```python
from build123d import *

# Parameters (mm, degrees)
CYLINDER017_R     = 3.5
CYLINDER017_DEPTH = 4
CYLINDER015_R     = 1.65
CYLINDER015_DEPTH = 20
CYLINDER016_R     = 3.5
CYLINDER016_DEPTH = 4
CYLINDER014_R     = 1.65
CYLINDER014_DEPTH = 20
BOX001_W          = 95
BOX001_H          = 30
BOX001_DEPTH      = 5
CYLINDER010_R     = 24.8
CYLINDER010_DEPTH = 10


with BuildPart() as zylinder017:
    # Cylinder017 → Cylinder017 (new body)
    with BuildSketch(Plane.XY):
        Circle(CYLINDER017_R)
    extrude(amount=CYLINDER017_DEPTH)


with BuildPart() as screw02:
    # Cylinder015 → Cylinder015 (new body)
    with BuildSketch(Plane.XY):
        Circle(CYLINDER015_R)
    extrude(amount=CYLINDER015_DEPTH)

    # Fusion003: union Zylinder017
    add(zylinder017.part)


with BuildPart() as screw02_1:
    # Fusion003 placement: moved
    add(screw02.part.moved(Location((4, 57, 10))))


with BuildPart() as zylinder016:
    # Cylinder016 → Cylinder016 (new body)
    with BuildSketch(Plane.XY):
        Circle(CYLINDER016_R)
    extrude(amount=CYLINDER016_DEPTH)


with BuildPart() as compound002:
    # Cylinder014 → Cylinder014 (new body)
    with BuildSketch(Plane.XY):
        Circle(CYLINDER014_R)
    extrude(amount=CYLINDER014_DEPTH)

    # Fusion002: union Zylinder016
    add(zylinder016.part)


with BuildPart() as compound002_1:
    # Fusion002 placement: moved
    add(compound002.part.moved(Location((4, 38, 10))))

    # Compound002: union Screw02
    add(screw02_1.part)


with BuildPart() as obj1:
    # Box001 → Box001 (new body)
    with BuildSketch(Plane(origin=(0, 32.5, 10), x_dir=(1, 0, 0), z_dir=(0, 0, 1))):
        with Locations((47.5, 15)):
            Rectangle(BOX001_W, BOX001_H)
    extrude(amount=BOX001_DEPTH)


with BuildPart() as rotatingtable:
    # Cylinder010 → Cylinder010 (new body)
    with BuildSketch(Plane(origin=(47.5, 47.5, 0), x_dir=(1, 0, 0), z_dir=(0, 0, 1))):
        Circle(CYLINDER010_R)
    extrude(amount=CYLINDER010_DEPTH)

    # Fusion001: union obj1
    add(obj1.part)

    # Cut006: cut Compound002
    add(compound002_1.part, mode=Mode.SUBTRACT)


solid = rotatingtable.part
```
Could you check a few things on this model? Use its own coordinates, in mm. A direction names the side the tool comes from. Give positions to 0.01 mm unless a question says otherwise; leave off trailing zeros. Order: outer loops, then holes, each group sorted by start corner. A loop starts at its lowest first (then second) coordinate and runs counter-clockwise, first axis right, second up.
Q1. Suppose I cut it at C-C, the plane z = 13. Write out the boundary of the cut face in (x, y), and give its area (3 significant figures).
Q2. Suppose I cut it at D-D, the plane x = 47.5. Write out the boundary of the cut face in (y, z), and give its area (3 significant figures).
Q3. For faces 1 (the flat face through (47, 32.5, 12)), 2 (the flat face through (47, 62.5, 12)), 3 (the cylindrical face through (7.34, 58.05, 11.97)), 4 (the flat face through (47, 48, 15)), which set-ups out of +Z, -Z, +X, -X, +Y, -Y let a thin tool reach every point of the face, with its end or its side?
Q4. Suppose I cut it at A-A, the plane x = 4. Write out the boundary of the cut face in (y, z), and give its area (3 significant figures).
Q5. I'm going to push flat-ended pins straight in: P1, Ø14, axis at x = 10, y = 48.5, coming from the -Z side; P2, Ø3, axis at x = 38.5, y = 28.5, coming from the +Z side; P3, Ø4, axis at x = 40, z = 11.5, coming from the +Y side. Where does each tip first touch, or does it pass through?
Q6. Suppose I cut it at B-B, the plane y = 38. Write out the boundary of the cut face in (x, z), and give its area (3 significant figures).
Q7. If I drill on line 1 along Y through (x, z) = (4, 14.4); line 2 along X through (y, z) = (57, 14.7); line 3 along Y through (x, z) = (4, 12.2), over which ranges is the centre line in solid material (lowest first)?
Solution:
1. outline: (0, 32.5) - (95, 32.5) - (95, 62.5) - (0, 62.5) - close; hole circle Ø7 at (4, 38); hole circle Ø7 at (4, 57)
1. area: 2,770 mm2
2. outline: (22.7, 0) - (72.3, 0) - (72.3, 10) - (62.5, 10) - (62.5, 15) - (32.5, 15) - (32.5, 10) - (22.7, 10) - close
2. area: 646 mm2
3. face 1: +Z, +X, -X, -Y
3. face 2: +Z, +X, -X, +Y
3. face 3: -Z
3. face 4: +Z, +X, -X, +Y, -Y
4. outline: (32.5, 10) - (34.5, 10) - (34.5, 14) - (36.35, 14) - (36.35, 15) - (32.5, 15) - close; (39.65, 14) - (41.5, 14) - (41.5, 10) - (53.5, 10) - (53.5, 14) - (55.35, 14) - (55.35, 15) - (39.65, 15) - close; (58.65, 14) - (60.5, 14) - (60.5, 10) - (62.5, 10) - (62.5, 15) - (58.65, 15) - close
4. area: 87.4 mm2
5. P1: stops at z = 10
5. P2: stops at z = 10
5. P3: stops at y = 71.52
6. outline: (0, 10) - (0.5, 10) - (0.5, 14) - (2.35, 14) - (2.35, 15) - (0, 15) - close; (5.65, 14) - (7.5, 14) - (7.5, 10) - (24.59, 10) - (24.59, 0) - (70.41, 0) - (70.41, 10) - (95, 10) - (95, 15) - (5.65, 15) - close
6. area: 902 mm2
7. line 1: y = 32.5 to 36.35, 39.65 to 55.35, 58.65 to 62.5
7. line 2: x = 0 to 2.35, 5.65 to 95
7. line 3: y = 32.5 to 34.5, 41.5 to 53.5, 60.5 to 62.5
